The model under review builds one solid part; all positions refer to its coordinate system, in mm. Face numbers are marked on the shaded views. A direction names the side the tool comes from. Round coordinates to 2 decimals unless told otherwise and drop trailing zeros. Loops run counter-clockwise (first coordinate to the right, second up) from the corner with the lowest first, then second, coordinate; pieces in that order, holes last. Notation, with made-up numbers: (31, 65.25) - (44, 65.25) arc R28 ccw to (44, 86.25) - close; hole circle Ø1 at (85, -17). An arc over 180 degrees is marked (long way). Answer as CSV lines item,"result".
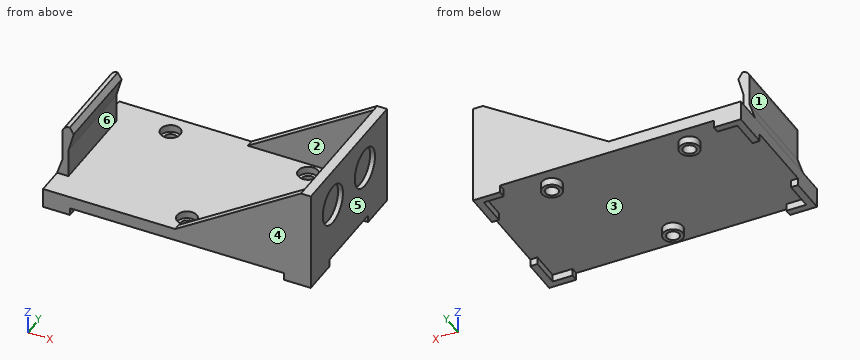
from build123d import *

# Parameters (mm, degrees)
SKETCH_W                = 54.5
SKETCH_H                = 30.2
PAD_DEPTH               = 2.5
PAD001_DEPTH            = 16.5
POCKET_DEPTH            = 30.201
PAD002_DEPTH            = 24.6
SKETCH004_W             = 5.6
SKETCH004_H             = 11
POCKET001_DEPTH         = 5
SKETCH005_R             = 2
PAD003_DEPTH            = 4
SKETCH006_R             = 2
POCKET002_DEPTH         = 1.5
SKETCH007_R             = 1.3
POCKET003_DEPTH         = 4.001
PAD004_DEPTH            = 1.5
PAD004_MIRRORED_2_DEPTH = 1.5
SKETCH012_R             = 4
POCKET006_DEPTH         = 1


with BuildPart() as part:
    # Sketch → Pad (new body)
    with BuildSketch(Plane.XY):
        Rectangle(SKETCH_W, SKETCH_H)
    extrude(amount=PAD_DEPTH)

    # Sketch001 (on Face6 of Pad) → Pad001 (join)
    with BuildSketch(Plane.XY.offset(2.5)):
        Polygon((27.25, 15.1), (27.25, -15.1), (-0.35, -15.1), (-0.35, -13.65), (25.25, -13.65), (25.25, 13.65), (-0.35, 13.65), (-0.35, 15.1), align=None)
    extrude(amount=PAD001_DEPTH)

    # Sketch002 (on Face15 of Pad001) → Pocket (cut, through all)
    with BuildSketch(Plane.XZ.offset(15.1)):
        Polygon((-0.35, 2.5), (25.25, 19), (27.25, 19), (27.25, 21), (-0.35, 21), align=None)
    extrude(amount=-POCKET_DEPTH, mode=Mode.SUBTRACT)

    # Sketch003 (on Face7 of Pocket) → Pad002 (join)
    with BuildSketch(Plane.XZ.offset(15.1)):
        with BuildLine():
            Line((-27.25, 2.5), (-26.177765, 5.8))
            Line((-26.177765, 5.8), (-26.177765, 12))
            ThreePointArc((-24.677765, 13.5), (-25.738425, 13.06066), (-26.177765, 12))
            Line((-24.677765, 13.5), (-23.877765, 12.2))
            Line((-23.877765, 12.2), (-24.95, 8.3))
            Line((-24.95, 8.3), (-24.95, 2.5))
            Line((-24.95, 2.5), (-27.25, 2.5))
        make_face()
    extrude(amount=-PAD002_DEPTH)

    # Sketch004 (on Face2 of Pad002) → Pocket001 (cut)
    with BuildSketch(Plane(origin=(-27.25, 0, 0), x_dir=(0, -1, 0), z_dir=(-1, 0, 0))):
        with Locations((12.3, 8)):
            Rectangle(SKETCH004_W, SKETCH004_H)
    extrude(amount=-POCKET001_DEPTH, mode=Mode.SUBTRACT)

    # Sketch005 (on Face5 of Pocket001) → Pad003 (join)
    with BuildSketch(Plane.XY.offset(2.5)):
        with Locations((-14.75, 11.1)):
            Circle(SKETCH005_R)
        with Locations((13.25, 11.1)):
            Circle(SKETCH005_R)
        with Locations((0, -11.1)):
            Circle(SKETCH005_R)
    extrude(amount=-PAD003_DEPTH)

    # Sketch006 (on Face5 of Pad003) → Pocket002 (cut)
    with BuildSketch(Plane.XY.offset(2.5)):
        with Locations((-14.75, 11.1)):
            Circle(SKETCH006_R)
        with Locations((13.25, 11.1)):
            Circle(SKETCH006_R)
        with Locations((0, -11.1)):
            Circle(SKETCH006_R)
    extrude(amount=-POCKET002_DEPTH, mode=Mode.SUBTRACT)

    # Sketch007 (on Face5 of Pocket002) → Pocket003 (cut, through all)
    with BuildSketch(Plane.XY.offset(2.5)):
        with Locations((-14.75, 11.1)):
            Circle(SKETCH007_R)
        with Locations((13.25, 11.1)):
            Circle(SKETCH007_R)
        with Locations((0, -11.1)):
            Circle(SKETCH007_R)
    extrude(amount=-POCKET003_DEPTH, mode=Mode.SUBTRACT)

    # Sketch008 (on Face4 of Pocket003) → Pad004 (join)
    with BuildSketch(Plane(origin=(0, 0, 0), x_dir=(1, 0, 0), z_dir=(0, 0, -1))):
        Polygon((-27.25, 15.1), (-21.75, 15.1), (-21.75, 13.65), (-25.8, 13.65), (-25.8, 7.6), (-27.25, 7.6), align=None)
    pad004 = extrude(amount=PAD004_DEPTH)

    # Sketch008 Mirrored 2 → Pad004 Mirrored 2 (add)
    with BuildSketch(Plane(origin=(0, 0, 0), x_dir=(-1, 0, 0), z_dir=(0, 0, 1))):
        Polygon((-27.25, 15.1), (-21.75, 15.1), (-21.75, 13.65), (-25.8, 13.65), (-25.8, 7.6), (-27.25, 7.6), align=None)
    pad004_mirrored_2 = extrude(amount=-PAD004_MIRRORED_2_DEPTH)

    # Mirrored001: Pad004, Pad004 Mirrored 2 across Sketch008 H_Axis
    add(pad004.mirror(Plane(origin=(0, 0, 0), x_dir=(0, 0, -1), z_dir=(0, -1, 0))))
    add(pad004_mirrored_2.mirror(Plane(origin=(0, 0, 0), x_dir=(0, 0, -1), z_dir=(0, -1, 0))))

    # Sketch012 (on Face16 of MultiTransform) → Pocket006 (cut)
    with BuildSketch(Plane.YZ.offset(27.25)):
        with Locations((-6.35, 11.5)):
            Circle(SKETCH012_R)
        with Locations((6.35, 11.5)):
            Circle(SKETCH012_R)
    extrude(amount=-POCKET006_DEPTH, mode=Mode.SUBTRACT)


solid = part.part
1. Take a section at B-B (y = 11.1). State how many separate pieces and enclosed holes the cut face has, plus the area to 3 significant figures.
Numbers:
separate pieces,"3"
enclosed holes,"0"
area,"161 mm²"
2. Tool access review of the marked faces 1, 2 and 3: name each direction out of +Z, -Z, +X, -X, +Y, -Y from which nothing blocks a thin tool from reaching the whole face with its end or side.
Numbers:
face 1,"+Z, -X, +Y, -Y"
face 2,"+Z, -X"
face 3,"-Z"
3. Take a section at C-C (y = -11.1). State the section outline as (x, z) points, plus the area to 3 significant figures.
Numbers:
outline,"(-27.25, -1.5) - (-25.8, -1.5) - (-25.8, 0) - (-2, 0) - (-2, -1.5) - (-1.3, -1.5) - (-1.3, 1) - (-2, 1) - (-2, 2.5) - (-27.25, 2.5) - close; (1.3, -1.5) - (2, -1.5) - (2, 0) - (25.8, 0) - (25.8, -1.5) - (27.25, -1.5) - (27.25, 19) - (25.25, 19) - (25.25, 2.5) - (2, 2.5) - (2, 1) - (1.3, 1) - close"
area,"167 mm²"
4. Wall thickness on probe 1 along Z at (x, y) = (26.6, 6.35); probe 2 along Y at (x, z) = (13.25, 2); probe 3 along Y at (x, z) = (0, 1.65): over which ranges is each line inside the solid? List them lowest first.
Numbers:
probe 1,"z = 0 to 7.5, 15.5 to 19"
probe 2,"y = -15.1 to 9.1, 13.1 to 15.1"
probe 3,"y = -15.1 to -13.1, -9.1 to 15.1"
5. Take a section at D-D (y = -6.35). State the section outline as (x, z) points, plus the area to 3 significant figures.
Numbers:
outline,"(-27.25, 0) - (27.25, 0) - (27.25, 7.5) - (26.25, 7.5) - (26.25, 15.5) - (27.25, 15.5) - (27.25, 19) - (25.25, 19) - (25.25, 2.5) - (-24.95, 2.5) - (-24.95, 8.3) - (-23.88, 12.2) - (-24.68, 13.5) arc R1.5 ccw to (-26.18, 12) - (-26.18, 5.8) - (-27.25, 2.5) - close"
area,"179 mm²"
6. Take a section at A-A (x = -14.75). State the section outline as (y, z) points.
Numbers:
outline,"(-15.1, 0) - (9.1, 0) - (9.1, -1.5) - (9.8, -1.5) - (9.8, 1) - (9.1, 1) - (9.1, 2.5) - (-15.1, 2.5) - close; (12.4, -1.5) - (13.1, -1.5) - (13.1, 0) - (15.1, 0) - (15.1, 2.5) - (13.1, 2.5) - (13.1, 1) - (12.4, 1) - close"
7. Draft analysis for pull direction X (two halves, no side actions). For the marked faces 4, 5 and 6, state which applies: +X half, -X half, draft (parallel to the pull), parting line (faces both ways), or undercut.
Numbers:
face 4,"draft"
face 5,"+X half"
face 6,"undercut"
8. Clearance check with flat-ended pins moving along their axes: pin 1 (4 mm diameter, centred on y = 5.5, z = 11, fed in from +X); pin 2 (3.5 mm diameter, centred on x = -25, z = 9, fed in from +Y); pin 3 (2.5 mm diameter, centred on x = 13.25, y = 11.1, fed in from +Z); pin 4 (1.9 mm diameter, centred on y = -3.5, z = 8.5, fed in from -X). State where each tip first meets the part, or that it passes through.
Numbers:
pin 1,"stops at x = 26.25"
pin 2,"stops at y = 9.5"
pin 3,"passes through"
pin 4,"stops at x = -26.18"
